```python
from build123d import *

# Parameters (mm, degrees)
F1_DEPTH = 3.175


with BuildPart() as f1:
    # F0 (on Front) → F1 (new body, symmetric)
    with BuildSketch(Plane.XZ):
        with BuildLine():
            Line((-311.3615883296, -165.1), (-263.9645430735, -165.1))
            ThreePointArc((-263.9645430735, -165.1), (-276.2318010674, -155.6870018728), (-270.3145430735, -141.4014773719))
            Line((-270.3145430735, -141.4014773719), (-311.3615883296, -165.1))
        make_face()
        with BuildLine():
            ThreePointArc((-257.6145430735, -163.3985226281), (-252.9660204454, -158.75), (-251.2645430735, -152.4))
            Line((-251.2645430735, -152.4), (-262.3770430735, -152.4))
            ThreePointArc((-262.3770430735, -152.4), (-265.4979503227, -152.8108752341), (-262.589727745, -151.60625))
            Line((-262.589727745, -151.60625), (-252.9660204454, -146.05))
            ThreePointArc((-252.9660204454, -146.05), (-257.6145430735, -141.4014773719), (-263.9645430735, -139.7))
            ThreePointArc((-263.9645430735, -139.7), (-267.2515449463, -140.1327420061), (-270.3145430735, -141.4014773719))
            ThreePointArc((-270.3145430735, -141.4014773719), (-276.2318010674, -155.6870018728), (-263.9645430735, -165.1))
            ThreePointArc((-263.9645430735, -165.1), (-260.6775412007, -164.6672579939), (-257.6145430735, -163.3985226281))
        make_face()
        with BuildLine():
            Line((-262.3770430735, -152.4), (-251.2645430735, -152.4))
            ThreePointArc((-251.2645430735, -152.4), (-251.6972850796, -149.1129981272), (-252.9660204454, -146.05))
            Line((-252.9660204454, -146.05), (-262.589727745, -151.60625))
            ThreePointArc((-262.589727745, -151.60625), (-262.4311358243, -151.9891247659), (-262.3770430735, -152.4))
        make_face()
        with BuildLine():
            Line((-238.5645430735, -152.4), (-251.2645430735, -152.4))
            ThreePointArc((-251.2645430735, -152.4), (-252.9660204454, -158.75), (-257.6145430735, -163.3985226281))
            Line((-257.6145430735, -163.3985226281), (-238.5645430735, -152.4))
        make_face()
        with BuildLine():
            ThreePointArc((-263.9645430735, -139.7), (-257.6145430735, -141.4014773719), (-252.9660204454, -146.05))
            Line((-252.9660204454, -146.05), (-241.9674978174, -139.7))
            Line((-241.9674978174, -139.7), (-263.9645430735, -139.7))
        make_face()
        with BuildLine():
            ThreePointArc((-252.9660204454, -146.05), (-251.6972850796, -149.1129981272), (-251.2645430735, -152.4))
            Line((-251.2645430735, -152.4), (-238.5645430735, -152.4))
            Line((-238.5645430735, -152.4), (-216.5674978174, -139.7))
            Line((-216.5674978174, -139.7), (-241.9674978174, -139.7))
            Line((-241.9674978174, -139.7), (-252.9660204454, -146.05))
        make_face()
        Polygon((-216.5674978174, -139.7), (-238.5645430735, -152.4), (-171.6615883296, -152.4), (-158.9615883296, -139.7), align=None)
        with BuildLine():
            Line((-171.6615883296, -152.4), (-238.5645430735, -152.4))
            Line((-238.5645430735, -152.4), (-257.6145430735, -163.3985226281))
            ThreePointArc((-257.6145430735, -163.3985226281), (-260.6775412007, -164.6672579939), (-263.9645430735, -165.1))
            Line((-263.9645430735, -165.1), (-158.9615883296, -165.1))
            Line((-158.9615883296, -165.1), (-171.6615883296, -152.4))
        make_face()
    extrude(amount=F1_DEPTH, both=True)


solid = f1.part
```
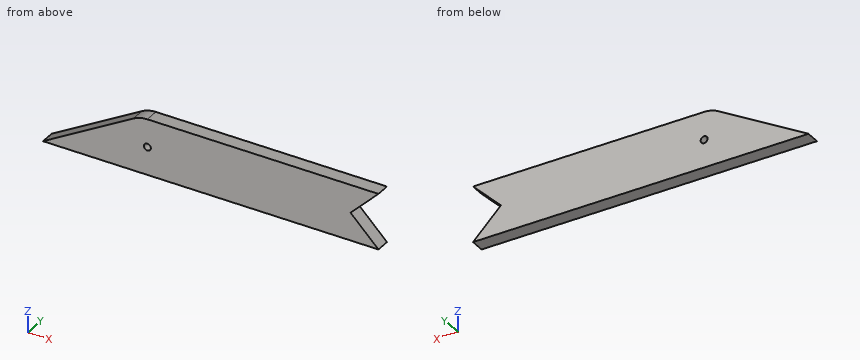
Verification items for the finished model (mm, model axes). Give positions to 0.01 mm unless a question says otherwise; leave off trailing zeros. Order: outer loops, then holes, each group sorted by start corner. A loop starts at its lowest first (then second) coordinate and runs counter-clockwise, first axis right, second up. Notation, with made-up numbers: (38, 52.25) - (50, 52.25) arc R33 cw to (50, 82.25) - close; hole circle Ø4 at (0.25, -18.5). An arc over 180 degrees is marked (long way). Answer as CSV lines item,"result". Start each with the question number.
Item 1: Gauge pin test, flat ends, axial feed: pin 1 (3.5 mm diameter, centred on x = -263.96, z = -152.4, fed in from -Y) (3 decimals); pin 2 (1 mm diameter, centred on y = -1, z = -155, fed in from +X); pin 3 (1 mm diameter, centred on y = -1.5, z = -148.5, fed in from +X). Record the tip position at first contact, or that the pin passes through.
Item 2: Section check B-B, the plane z = -155.5. Record the boundary of the cut face in (x, y) (3 decimals), plus the area to 3 significant figures.
Item 3: Section check A-A, the plane x = -272. Record the boundary of the cut face in (y, z) (3 decimals).
Item 4: Material ranges on L1, parallel to Z at x = -164.5, y = -1; L2, parallel to X at y = -1, z = -151.5; L3, parallel to X at y = 1.5, z = -152.4, recorded low to high.
Filled in:
1,pin 1,"y = -3.175"
1,pin 2,"x = -168.56"
1,pin 3,"x = -167.26"
2,outline,"(-294.734, -3.175) - (-168.562, -3.175) - (-168.562, 3.175) - (-294.734, 3.175) - close"
2,area,"801 mm^2"
3,outline,"(-3.175, -165.1) - (3.175, -165.1) - (3.175, -142.375) - (-3.175, -142.375) - close"
4,L1,"-165.1 to -159.56, -145.24 to -139.7"
4,L2,"-287.81 to -265.27, -262.66 to -170.76"
4,L3,"-289.36 to -265.55, -262.38 to -171.66"
